Design review of the part built by this model. Coordinates are the model's own, in mm. A direction names the side the tool comes from. Coordinates: 2 decimals unless noted, no trailing zeros. Loops run counter-clockwise (first coordinate to the right, second up) from the corner with the lowest first, then second, coordinate; pieces in that order, holes last. Notation, with made-up numbers: M -15.75,-19.5 L 37.25,-19.5 A14 cw 37.25,6.5 Z; hole C -27,48.5 d10. An arc over 180 degrees is marked long. Answer as a JSON object with one key per item and string values. Group by question number.
1. Consider section D-D (z = -12.5). Count the separate pieces of the cut face and the enclosed holes in it, then the cut area to 3 significant figures.
2. Consider section C-C (x = 34). State the section outline as (y, z) points (1 decimal).
3. Consider section A-A (y = 8.5). State the section outline as (x, z) points (3 decimals), then the cut area to 3 significant figures.
4. Draft analysis for pull direction X (two halves, no side actions). For faces 1 (the flat face through (-12.31, 21.57, 15.85)), 2 (the flat face through (-13.081, 17, 16)), 3 (the cylindrical face through (57.696, 11.734, 22.731)), state which applies: +X half, -X half, draft (parallel to the pull), parting line (faces both ways), or undercut.
5. Consider section B-B (z = -0.5). State the section outline as (x, y) points, then the cut area to 3 significant figures.
6. Insertion check: pin 1 (5 mm diameter, centred on y = 16.5, z = -15.5, fed in from +X); pin 2 (2 mm diameter, centred on y = 13.5, z = -13, fed in from +X); pin 3 (0.6 mm diameter, centred on y = 11.5, z = 24, fed in from +X); pin 4 (6.5 mm diameter, centred on x = -9.5, y = 19.5, fed in from +Z). Each pin has a flat end and moves straight along its axis. Give the tip position at first contact, or say it passes through.
7. Machinability: for faces 4 (the flat face through (58, 10.795, 23)), 5 (the flat face through (0.762, 17, -16)), 6 (the flat face through (37.16, 21.61, -15.71)), 7 (the cylindrical face through (57.656, 11.734, -22.771)), 8 (the flat face through (11.557, 17, 16)), which of the approach directions +Z, -Z, +X, -X, +Y, -Y give a long, thin tool a straight path to every point of the face, cutting with its end or side? Answer none if there is none.
8. To check wall thickness, follow probe 1 along X at (y, z) = (12.5, -15); probe 2 along Z at (x, y) = (-50, 10) (3 decimals); probe 3 along Z at (x, y) = (47.5, 5) (3 decimals). State the ranges of each line that lie inside material, in increasing order.
Autodesk Inventor part; units mm, degrees
ref_plane "YZ Plane" through (0, 0, 0) normal (1, 0, 0) x (0, 1, 0)
ref_plane "XZ Plane" through (0, 0, 0) normal (0, 1, 0) x (-1, 0, 0)
ref_plane "XY Plane" through (0, 0, 0) normal (0, 0, 1) x (1, 0, 0)
sketch "Sketch1" plane through (0, 0, 0) normal (0, 1, 0) x (-1, 0, 0)
  line L0 (59.69, -24.765) -> (-59.69, -24.765)
  line L1 (-59.69, -24.765) -> (-59.69, 24.765)
  line L2 (-59.69, 24.765) -> (59.69, 24.765)
  line L3 (59.69, 24.765) -> (59.69, -24.765)
  line L4 (59.69, -24.765) -> (-59.69, 24.765) construction
  line L5 (-59.69, -24.765) -> (59.69, 24.765) construction
  point P0 (0, 0)
  dimension "d0" = 119.38
  dimension "d1" = 59.69
  dimension "d2" = 49.53
  dimension "d3" = 24.765
extrude "Extrusion1" add sketch "Sketch1" along normal blind 12.7
sketch "Sketch2" plane through (0, 12.7, 0) normal (0, 1, 0) x (1, 0, 0)
  line L0 (38.1, -23.495) -> (-38.1, -23.495)
  line L1 (-38.1, -23.495) -> (-38.1, 23.495)
  line L2 (-38.1, 23.495) -> (38.1, 23.495)
  line L3 (38.1, 23.495) -> (38.1, -23.495)
  line L4 (59.69, -24.765) -> (59.69, 24.765)
  line L5 (-59.69, -24.765) -> (59.69, -24.765)
  line L6 (-59.69, 24.765) -> (-59.69, -24.765)
  point P0 (0, 0)
  dimension "d6" = 21.59
  dimension "d7" = 76.2
  dimension "d8" = 1.27
  dimension "d9" = 46.99
  dimension "d10" = 21.59
extrude "Extrusion2" add sketch "Sketch2" along normal blind 12.7
sketch "Sketch3" plane through (0, 25.4, 0) normal (0, 1, 0) x (1, 0, 0)
  line L0 (-38.1, 23.495) -> (38.1, 23.495)
  line L1 (36.195, 23.495) -> (25.4, 23.495)
  line L2 (25.4, 23.495) -> (25.4, 11.1125)
  line L3 (25.4, 11.1125) -> (36.195, 11.1125)
  line L4 (36.195, 11.1125) -> (36.195, 23.495)
  line L5 (38.1, -23.495) -> (38.1, 23.495)
  point P0 (0, 0)
  dimension "d13" = 1.905
  dimension "d14" = 10.795
  dimension "d15" = 11.1125
extrude "Extrusion3" cut sketch "Sketch3" against normal up to surface (12.7 mm away)
pattern_linear "Rectangular Pattern1" count 6 spacing 12.319 along (-1, 0, 0) count 2 spacing -34.6075 along (0, 0, -1) of "Extrusion3"
sketch "Sketch4" plane through (0, 12.7, 0) normal (0, 1, 0) x (1, 0, 0)
  line L0 (-59.69, 24.765) -> (-59.69, -24.765)
  line L1 (-59.69, -15.113) -> (-58.42, -15.113)
  line L2 (-58.42, -15.113) -> (-58.42, -23.495)
  line L3 (-58.42, -23.495) -> (-50.038, -23.495)
  line L4 (-50.038, -23.495) -> (-50.038, -24.765)
  line L5 (-50.038, -24.765) -> (-59.69, -24.765)
  line L6 (-59.69, -24.765) -> (-59.69, -15.113)
  line L7 (-59.69, 24.765) -> (-59.69, 15.113)
  line L8 (-59.69, 15.113) -> (-58.42, 15.113)
  line L9 (-58.42, 15.113) -> (-58.42, 23.495)
  line L10 (-58.42, 23.495) -> (-50.038, 23.495)
  line L11 (-50.038, 23.495) -> (-50.038, 24.765)
  line L12 (-50.038, 24.765) -> (-59.69, 24.765)
  point P0 (0, 0)
  dimension "d24" = 1.27
  dimension "d25" = 1.27
  dimension "d26" = 8.382
  dimension "d27" = 1.27
  dimension "d28" = 1.27
extrude "Extrusion4" cut sketch "Sketch4" against normal blind 1.905
mirror "Mirror1" about plane through (0, 0, 0) normal (1, 0, 0) of "Extrusion4"
sketch "Sketch5" plane through (0, 12.7, 0) normal (0, 1, 0) x (1, 0, 0)
  line L0 (-50.038, -24.765) -> (50.038, -24.765)
  line L1 (59.69, -15.113) -> (59.69, 15.113)
  line L2 (50.038, 24.765) -> (-50.038, 24.765)
  point P0 (0, 0)
  point P1 (50.038, -15.113)
  point P2 (50.038, 15.113)
  dimension "d38" = 9.652
  dimension "d39" = 9.652
  dimension "d40" = 9.652
  dimension "d41" = 9.652
hole "Hole1" at (50.038, 12.7, 15.113) at (50.038, 12.7, -15.113) direction (0, -1, 0) diameter 7.62 end through all
mirror "Mirror2" about plane through (0, 0, 0) normal (1, 0, 0) of "Hole1"
fillet "Fillet1" radius 3.81 4 edges at (59.69, 5.3975, -24.765) (59.69, 5.3975, 24.765) (-59.69, 5.3975, 24.765) (-59.69, 5.3975, -24.765)
fillet "Fillet1" radius 2.54 4 edges at (-58.42, 11.7475, -23.495) (-58.42, 11.7475, 23.495) (58.42, 11.7475, -23.495) (58.42, 11.7475, 23.495)
sketch "Sketch6" plane through (38.1, 12.7, 23.495) normal (1, 0, 0) x (0, 0, -1)
  line L0 (0, 0) -> (0, 12.7)
  line L1 (0, 0) -> (3.048, 7.62)
  line L2 (46.99, 12.7) -> (0, 12.7)
  line L3 (0, 12.7) -> (12.3825, 12.7)
  line L4 (0, 12.7) -> (0, 0)
  line L5 (2.54, 0) -> (8.382, 0)
  line L6 (3.048, 7.62) -> (12.3825, 10.16)
  line L7 (12.3825, 10.16) -> (12.3825, 12.7)
  point P0 (23.495, -12.7)
  point P1 (12.3825, 12.7)
  dimension "d44" = 7.62
  dimension "d45" = 12.3825
  dimension "d46" = 2.54
  dimension "d47" = 2.54
  dimension "d49" = 3.048
extrude "Extrusion5" cut sketch "Sketch6" against normal through all
mirror "Mirror3" about plane through (0, 0, 0) normal (0, 0, 1) of "Extrusion5"
properties part number "CO-1-01-12VoltFuse"
Findings below:
{
 "1": {"separate pieces": "3", "enclosed holes": "0", "area": "1,490 mm^2"},
 "2": {"outline": "M 0,-24.8 L 12.7,-24.8 L 12.7,-11.1 L 25.4,-11.1 L 25.4,11.1 L 12.7,11.1 L 12.7,24.8 L 0,24.8 Z"},
 "3": {"outline": "M -59.69,-20.955 A3.81 ccw -55.88,-24.765 L 55.88,-24.765 A3.81 ccw 59.69,-20.955 L 59.69,20.955 A3.81 ccw 55.88,24.765 L -55.88,24.765 A3.81 ccw -59.69,20.955 Z; hole C -50.038,-15.113 d7.62; hole C -50.038,15.113 d7.62; hole C 50.038,-15.113 d7.62; hole C 50.038,15.113 d7.62", "area": "5,720 mm^2"},
 "4": {"face 1": "draft", "face 2": "undercut", "face 3": "+X half"},
 "5": {"outline": "M -59.69,0 L 59.69,0 L 59.69,12.7 L 38.1,12.7 L 38.1,25.4 L -38.1,25.4 L -38.1,12.7 L -59.69,12.7 Z", "area": "2,480 mm^2"},
 "6": {"pin 1": "stops at x = 38.1", "pin 2": "stops at x = 59.69", "pin 3": "stops at x = 50.04", "pin 4": "stops at z = 21.78"},
 "7": {"face 4": "+Z, +X, +Y", "face 5": "-Z, +Y", "face 6": "-Z, +X, -X, +Y", "face 7": "-Z, +X, +Y", "face 8": "+Z, +Y"},
 "8": {"probe 1": "x = -59.69 to -53.85, -46.23 to 46.23, 53.85 to 59.69", "probe 2": "z = -24.765 to -18.923, -11.303 to 11.303, 18.923 to 24.765", "probe 3": "z = -24.765 to -17.955, -12.271 to 12.271, 17.955 to 24.765"}
}
